Source: CAD feature listing. Evaluate the final solid. Frame: model axes, mm. Face numbers are marked on the shaded views. A direction names the side the tool comes from. Round coordinates to 2 decimals unless told otherwise and drop trailing zeros. Loops run counter-clockwise (first coordinate to the right, second up) from the corner with the lowest first, then second, coordinate; pieces in that order, holes last. Notation, with made-up numbers: M 42,41.5 L 91,41.5 A9 ccw 91,50.5 Z; hole C 36,82.5 d7. An arc over 180 degrees is marked long. Answer as a JSON object with one key per item and string values.
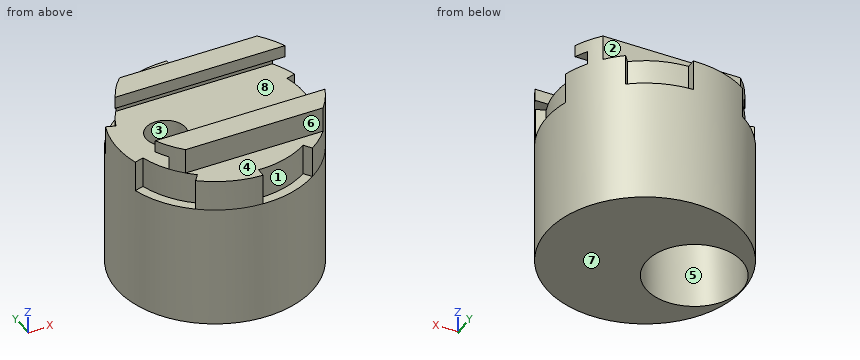
from build123d import *

# Parameters (mm, degrees)
SKETCH1_R           = 28.7
BOSS_EXTRUDE1_DEPTH = 50
SKETCH1_3_R         = 31.75
SKETCH1_3_R_2       = 28.7
BOSS_EXTRUDE2_DEPTH = 40
SKETCH3_R           = 6.375
CUT_EXTRUDE1_DEPTH  = 50
SKETCH3_3_R         = 15.5
SKETCH3_3_R_2       = 6.375
CUT_EXTRUDE2_DEPTH  = 25
BOSS_EXTRUDE3_START = -10
BOSS_EXTRUDE3_DEPTH = 10
BOSS_EXTRUDE4_DEPTH = 30
SKETCH7_OUTSIDE_W   = 86.902
SKETCH7_OUTSIDE_H   = 86.902
CUT_EXTRUDE3_DEPTH  = 68.202120502


# Read off the part's stored shape, not the designer's step: Boss-Extrude3
with BuildPart() as part:
    # Sketch1 → Boss-Extrude1 (new body)
    with BuildSketch(Plane.XY):
        Circle(SKETCH1_R)
    extrude(amount=BOSS_EXTRUDE1_DEPTH)

    # Sketch1<3> → Boss-Extrude2 (add)
    with BuildSketch(Plane.XY):
        Circle(SKETCH1_3_R)
        Circle(SKETCH1_3_R_2, mode=Mode.SUBTRACT)
    extrude(amount=BOSS_EXTRUDE2_DEPTH)

    # Sketch3 → Cut-Extrude1 (cut)
    with BuildSketch(Plane(origin=(0, 0, 0), x_dir=(-1, 0, 0), z_dir=(0, 0, -1))):
        with Locations((16, 0)):
            Circle(SKETCH3_R)
    extrude(amount=-CUT_EXTRUDE1_DEPTH, mode=Mode.SUBTRACT)

    # Sketch3<3> → Cut-Extrude2 (cut)
    with BuildSketch(Plane(origin=(0, 0, 0), x_dir=(-1, 0, 0), z_dir=(0, 0, -1))):
        with Locations((16, 0)):
            Circle(SKETCH3_3_R)
        with Locations(Location((16, 0, 0), (0, 0, 180))):
            Circle(SKETCH3_3_R_2, mode=Mode.SUBTRACT)
    extrude(amount=-CUT_EXTRUDE2_DEPTH, mode=Mode.SUBTRACT)

    # Boss-Extrude3 outline → Boss-Extrude3 (add)
    with BuildSketch(Plane.XY.offset(50).offset(BOSS_EXTRUDE3_START)):
        with BuildLine():
            Line((-30.520058846, -8.751486047), (-27.588210673, -7.910792112))
            ThreePointArc((-27.588210673, -7.910792112), (-28.682516735, 1.001615555), (-26.969178217, 9.815978113))
            Line((-26.969178217, 9.815978113), (-29.83524071, 10.859139551))
            ThreePointArc((-29.83524071, 10.859139551), (-31.730658758, 1.108059021), (-30.520058846, -8.751486047))
        make_face()
        with BuildLine():
            ThreePointArc((-1.001615555, -28.682516735), (-9.815978113, -26.969178217), (-17.669484342, -22.615908629))
            Line((-17.669484342, -22.615908629), (-19.547251842, -25.019341427))
            ThreePointArc((-19.547251842, -25.019341427), (-10.859139551, -29.83524071), (-1.10805902, -31.730658758))
            Line((-1.10805902, -31.730658758), (-1.001615555, -28.682516735))
        make_face()
        with BuildLine():
            Line((-17.754374685, 26.321942929), (-16.04883633, 23.793378332))
            ThreePointArc((-16.04883633, 23.793378332), (-7.910792112, 27.588210673), (1.001615555, 28.682516735))
            Line((1.001615555, 28.682516735), (1.10805902, 31.730658758))
            ThreePointArc((1.10805902, 31.730658758), (-8.751486047, 30.520058846), (-17.754374685, 26.321942929))
        make_face()
        with BuildLine():
            ThreePointArc((26.969178217, -9.815978113), (22.615908629, -17.669484341), (16.04883633, -23.793378332))
            Line((16.04883633, -23.793378332), (17.754374685, -26.321942929))
            ThreePointArc((17.754374685, -26.321942929), (25.019341427, -19.547251842), (29.83524071, -10.859139551))
            Line((29.83524071, -10.859139551), (26.969178217, -9.815978113))
        make_face()
        with BuildLine():
            Line((19.547251842, 25.019341427), (17.669484342, 22.615908629))
            ThreePointArc((17.669484342, 22.615908629), (23.793378332, 16.04883633), (27.588210673, 7.910792112))
            Line((27.588210673, 7.910792112), (30.520058846, 8.751486047))
            ThreePointArc((30.520058846, 8.751486047), (26.321942929, 17.754374685), (19.547251842, 25.019341427))
        make_face()
    extrude(amount=BOSS_EXTRUDE3_DEPTH)

    # Sketch5 → Boss-Extrude4 (add, symmetric)
    with BuildSketch(Plane(origin=(0, 0, 0), x_dir=(0, 0, -1), z_dir=(1, 0, 0))):
        Polygon((-58.2, -12.3), (-54.3, -12.3), (-54.3, -16.3), (-50, -16.3), (-50, -20.3), (-58.2, -20.3), align=None)
    boss_extrude4 = extrude(amount=BOSS_EXTRUDE4_DEPTH, both=True)

    # Mirror1: Boss-Extrude4 across plane
    add(boss_extrude4.mirror(Plane.ZX))

    # Sketch7 outside → Cut-Extrude3 (cut, through all)
    with BuildSketch(Plane.XY.offset(50)):
        Rectangle(SKETCH7_OUTSIDE_W, SKETCH7_OUTSIDE_H)
        with BuildLine():
            Line((-17.669484342, -22.615908629), (-19.547251842, -25.019341427))
            ThreePointArc((-19.547251842, -25.019341427), (-10.859139551, -29.83524071), (-1.10805902, -31.730658758))
            Line((-1.10805902, -31.730658758), (-1.001615555, -28.682516735))
            ThreePointArc((-1.001615555, -28.682516735), (7.910792112, -27.588210673), (16.04883633, -23.793378332))
            Line((16.04883633, -23.793378332), (17.754374685, -26.321942929))
            ThreePointArc((17.754374685, -26.321942929), (25.019341427, -19.547251842), (29.83524071, -10.859139551))
            Line((29.83524071, -10.859139551), (26.969178217, -9.815978113))
            ThreePointArc((26.969178217, -9.815978113), (28.682516735, -1.001615555), (27.588210673, 7.910792112))
            Line((27.588210673, 7.910792112), (30.520058846, 8.751486047))
            ThreePointArc((30.520058846, 8.751486047), (26.321942929, 17.754374685), (19.547251842, 25.019341427))
            Line((19.547251842, 25.019341427), (17.669484342, 22.615908629))
            ThreePointArc((17.669484342, 22.615908629), (9.815978113, 26.969178217), (1.001615555, 28.682516735))
            Line((1.001615555, 28.682516735), (1.10805902, 31.730658758))
            ThreePointArc((1.10805902, 31.730658758), (-8.751486047, 30.520058846), (-17.754374685, 26.321942929))
            Line((-17.754374685, 26.321942929), (-16.04883633, 23.793378332))
            ThreePointArc((-16.04883633, 23.793378332), (-22.615908629, 17.669484342), (-26.969178217, 9.815978113))
            Line((-26.969178217, 9.815978113), (-29.83524071, 10.859139551))
            ThreePointArc((-29.83524071, 10.859139551), (-31.730658758, 1.10805902), (-30.520058846, -8.751486047))
            Line((-30.520058846, -8.751486047), (-27.588210673, -7.910792112))
            ThreePointArc((-27.588210673, -7.910792112), (-23.793378332, -16.04883633), (-17.669484342, -22.615908629))
        make_face(mode=Mode.SUBTRACT)
    extrude(amount=CUT_EXTRUDE3_DEPTH, mode=Mode.SUBTRACT)


solid = part.part
Item 1: Pull-direction query (Y, two-part tool) for the marked faces 6, 7 and 8; classes: pulls with the +Y half, pulls with the -Y half, needs draft (parallel to the pull), parting line crosses it, or undercut.
Answer sheet:
{"face 6": "pulls with the -Y half", "face 7": "needs draft", "face 8": "undercut"}
Item 2: Section A-A on z = 41. Return the cut outline in (x, y) (3 decimals), then the cut area to 3 significant figures.
Answer sheet:
{"outline": "M -30.52,-8.751 L -27.588,-7.911 A28.7 ccw -17.669,-22.616 L -19.547,-25.019 A31.75 ccw -1.108,-31.731 L -1.002,-28.683 A28.7 ccw 16.049,-23.793 L 17.754,-26.322 A31.75 ccw 29.835,-10.859 L 26.969,-9.816 A28.7 ccw 27.588,7.911 L 30.52,8.751 A31.75 ccw 19.547,25.019 L 17.669,22.616 A28.7 ccw 1.002,28.683 L 1.108,31.731 A31.75 ccw -17.754,26.322 L -16.049,23.793 A28.7 ccw -26.969,9.816 L -29.835,10.859 A31.75 ccw Z; hole C -16,0 d12.75", "area": "2,750 mm²"}
Item 3: Access query for the marked faces 1, 2, 3, 4 and 5. Directions: +Z, -Z, +X, -X, +Y, -Y. A direction counts if a zero-diameter tool reaches every point of the face in a straight line with its end or side. Return the directions, or none.
Answer sheet:
{"face 1": "+Z, -Y", "face 2": "+Z, +X, -X, +Y", "face 3": "+Z, -Z", "face 4": "+Z, +X, -X, -Y", "face 5": "-Z"}
Item 4: Section D-D on z = 5. Return the cut outline in (x, y).
Answer sheet:
{"outline": "C 0,0 d63.5; hole C -16,0 d31"}
Item 5: Section C-C on x = 3. Return the cut outline in (y, z).
Answer sheet:
{"outline": "M -31.61,0 L 31.61,0 L 31.61,40 L 28.54,40 L 28.54,50 L 20.3,50 L 20.3,58.2 L 12.3,58.2 L 12.3,54.3 L 16.3,54.3 L 16.3,50 L -16.3,50 L -16.3,54.3 L -12.3,54.3 L -12.3,58.2 L -20.3,58.2 L -20.3,50 L -28.54,50 L -28.54,40 L -31.61,40 Z"}
Item 6: Section B-B on y = 0. Return the cut outline in (x, z) (3 decimals).
Answer sheet:
{"outline": "M -31.75,0 L -31.5,0 L -31.5,25 L -22.375,25 L -22.375,50 L -31.75,50 Z; M -9.625,25 L -0.5,25 L -0.5,0 L 31.75,0 L 31.75,40 L 28.7,40 L 28.7,50 L -9.625,50 Z"}
Item 7: Contact query for flat-ended pins moving along their axis: pin 1 Ø2.5 at (x, y) = (8, -29) entering from +Z; pin 2 Ø1 at (x, z) = (-22, 38) entering from +Y; pin 3 Ø1 at (x, y) = (-8, -3) entering from +Z; pin 4 Ø7.5 at (x, y) = (-16, 0) entering from -Z. Output: stop coordinate, or through.
Answer sheet:
{"pin 1": "stops at z = 40", "pin 2": "stops at y = 23.36", "pin 3": "stops at z = 50", "pin 4": "passes through"}
Item 8: Line query: probe 1 along Z at (x, y) = (12, 14); probe 2 along X at (y, z) = (0, 31.75) (3 decimals); probe 3 along Y at (x, z) = (9, 54). Output: solid intervals per line, ascending. Write a range as from..to.
Answer sheet:
{"probe 1": "z = 0..50, 54.3..58.2", "probe 2": "x = -31.75..-22.375, -9.625..31.75", "probe 3": "y = -20.3..-16.3, 16.3..20.3"}
